from build123d import *

# Parameters (mm, degrees)
F0_W     = 152.4
F0_H     = 101.6
F1_DEPTH = 127
F2_W     = 63.5
F2_H     = 50.8
F3_DEPTH = 101.6
F5_R     = 14.379735
F6_DEPTH = 152.4


with BuildPart() as f1:
    # F0 (on Top) → F1 (new body)
    with BuildSketch(Plane.XY):
        with Locations((16.524124, 4.168936)):
            Rectangle(F0_W, F0_H)
    extrude(amount=F1_DEPTH)

    # F2 (on face) → F3 (cut)
    with BuildSketch(Plane.XZ.offset(46.631064)):
        with Locations((60.974124, 101.6)):
            Rectangle(F2_W, F2_H)
    extrude(amount=-F3_DEPTH, mode=Mode.SUBTRACT)

    # F5 (on face) → F6 (cut)
    with BuildSketch(Plane(origin=(-59.675876, 0, 0), x_dir=(0, -1, 0), z_dir=(-1, 0, 0))):
        with Locations((-4.168936, 38.1)):
            Circle(F5_R)
    extrude(amount=-F6_DEPTH, mode=Mode.SUBTRACT)


solid = f1.part
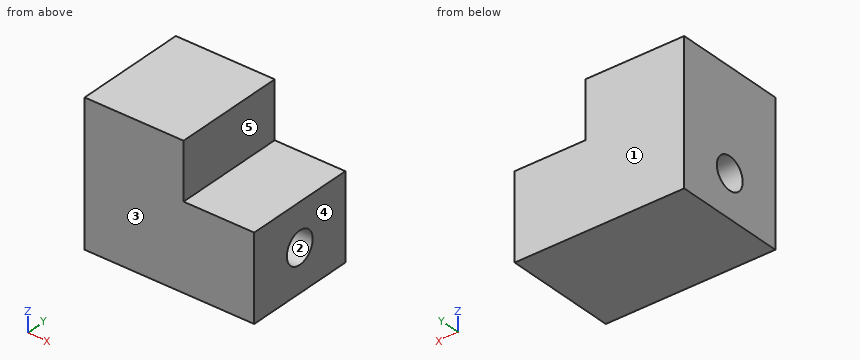
The listing builds one solid part. Answer for the finished solid, in the listing's coordinates (mm). Face numbers are marked on the shaded views. A direction names the side the tool comes from. Round coordinates to 2 decimals unless told otherwise and drop trailing zeros. Order: outer loops, then holes, each group sorted by start corner. A loop starts at its lowest first (then second) coordinate and runs counter-clockwise, first axis right, second up. Notation, with made-up numbers: (32, 35) -> (71, 35) arc R32 ccw to (71, 72) -> close; hole circle Ø9 at (-23, 8.25). An arc over 180 degrees is marked (long way). Put each result on its own line as item: value.
Q1. Section C-C, the plane y = 12 is taken. Write down the section's boundary in (x, z), and give its area (3 significant figures).
Results list:
outline: (-59.68, 0) -> (92.72, 0) -> (92.72, 26.04) -> (-59.68, 26.04) -> close; (-59.68, 50.16) -> (92.72, 50.16) -> (92.72, 76.2) -> (29.22, 76.2) -> (29.22, 127) -> (-59.68, 127) -> close
area: 12,500 mm^2
Q2. Consider line 1 along Y through (x, z) = (10, 38); line 2 along Z through (x, y) = (-31.5, 3.5); line 3 along Z through (x, y) = (47, -28). Determine where each line is inside the solid, lowest interval first.
Results list:
line 1: -46.63 to -10.21, 18.55 to 54.97
line 2: 0 to 23.74, 52.46 to 127
line 3: 0 to 76.2
Q3. Section D-D, the plane y = 45 is taken. Write down the section's boundary in (x, z), and give its area (3 significant figures).
Results list:
outline: (-59.68, 0) -> (92.72, 0) -> (92.72, 76.2) -> (29.22, 76.2) -> (29.22, 127) -> (-59.68, 127) -> close
area: 16,100 mm^2
Q4. Section B-B, the plane x = 56 is taken. Write down the section's boundary in (y, z), and give its area (3 significant figures).
Results list:
outline: (-46.63, 0) -> (54.97, 0) -> (54.97, 76.2) -> (-46.63, 76.2) -> close; hole circle Ø28.76 at (4.17, 38.1)
area: 7,090 mm^2
Q5. Which of the six approach directions +Z, -Z, +X, -X, +Y, -Y give full straight-line access (tool end or side, diameter ignored) to the marked faces 4 and 5?
Results list:
face 4: +Z, -Z, +X, +Y, -Y
face 5: +Z, +X, +Y, -Y
Q6. Determine the mould class of the marked faces 1, 2 and 3 for opening direction Y: pulls with the +Y half, pulls with the -Y half, needs draft (parallel to the pull), parting line crosses it, or undercut.
Results list:
face 1: pulls with the +Y half
face 2: undercut
face 3: pulls with the -Y half
Q7. Each of these flat-tipped pins is pushed along its axis until it touches: P1, Ø23, axis at y = 4.17, z = 38.1, coming from the +X side; P2, Ø8, axis at y = 42, z = 92.5, coming from the +X side; P3, Ø5, axis at x = 73.5, y = 12, coming from the +Z side. Where does it stop, or does it pass through?
Results list:
P1: through
P2: x = 29.22
P3: z = 76.2
Q8. Section A-A, the plane z = 38.1 is taken. Write down the section's boundary in (x, y).
Results list:
outline: (-59.68, -46.63) -> (92.72, -46.63) -> (92.72, -10.21) -> (-59.68, -10.21) -> close; (-59.68, 18.55) -> (92.72, 18.55) -> (92.72, 54.97) -> (-59.68, 54.97) -> close
